Check sheet for the drawn part. Datum: minimum x, y, z corner. Units: mm. Round coordinates to 2 decimals unless told otherwise and drop trailing zeros. Write each loop counter-clockwise with the first axis right and the second up, starting at its lowest first coordinate (ties: lowest second). Pieces come first, ordered by that corner, then holes.
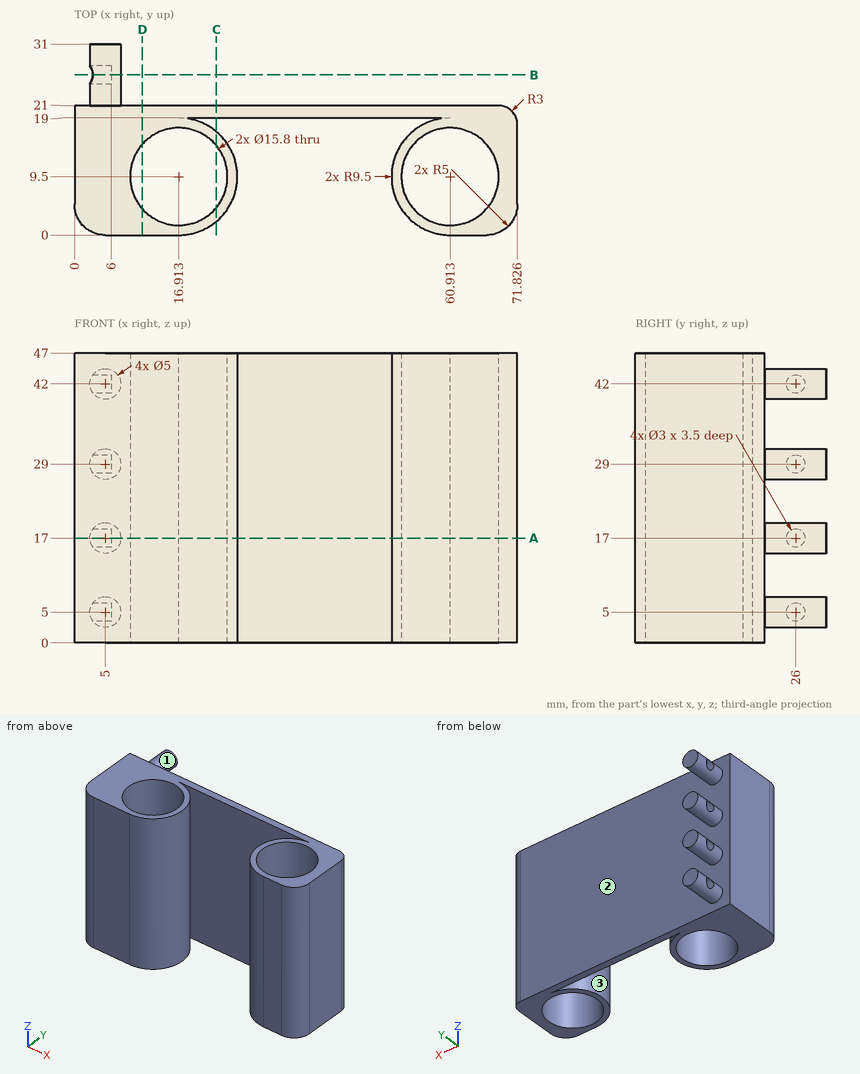
1. Sectioned sample at B-B, the plane y = 26. Enter the section's corners in (x, z).
2. Sectioned sample at D-D, the plane x = 11. Enter the section's corners in (y, z).
3. Release check for a two-part mould opening along Y. For the marked faces 1, 2 and 3 record: released by +Y, released by -Y, zero draft, split by the parting line, or undercut.
4. Scan lines: line 1 along X through (y, z) = (10, 34); line 2 along Y through (x, z) = (56, 24) (1 decimal); line 3 along Y through (x, z) = (5.2, 42). Record each from-to range of solid material in increasing order.
5. Go/stop test with flat-tipped pins: pin 1 (2.5 mm diameter, centred on y = 26, z = 42, fed in from +X); pin 2 (2.5 mm diameter, centred on y = 26, z = 5, fed in from -X); pin 3 (3.5 mm diameter, centred on y = 26, z = 5.5, fed in from -X); pin 4 (6 mm diameter, centred on x = 32, y = 23, fed in from -Z). Record where each tip stops, or that it passes through.
6. Sectioned sample at C-C, the plane x = 23. Enter the section's corners in (y, z).
7. Sectioned sample at A-A, the plane z = 17. Enter the section's corners in (x, y).
Computed values:
1. outline: (3, 3.5) arc R2.5 ccw (long way) to (3, 6.5) - (6, 6.5) - (6, 3.5) - close; (3, 15.5) arc R2.5 ccw (long way) to (3, 18.5) - (6, 18.5) - (6, 15.5) - close; (3, 27.5) arc R2.5 ccw (long way) to (3, 30.5) - (6, 30.5) - (6, 27.5) - close; (3, 40.5) arc R2.5 ccw (long way) to (3, 43.5) - (6, 43.5) - (6, 40.5) - close
2. outline: (0, 0) - (4.26, 0) - (4.26, 47) - (0, 47) - close; (14.74, 0) - (21, 0) - (21, 47) - (14.74, 47) - close
3. face 1: zero draft
3. face 2: released by +Y
3. face 3: undercut
4. line 1: x = 0 to 9.03, 24.8 to 26.4, 51.43 to 53.03, 68.8 to 71.83
4. line 2: y = 1.4 to 3.3, 15.7 to 17.6, 19 to 21
4. line 3: y = 0 to 24.5, 27.5 to 31
5. pin 1: stops at x = 7.5
5. pin 2: stops at x = 6
5. pin 3: stops at x = 2.5
5. pin 4: stops at z = 0
6. outline: (2.21, 0) - (4.46, 0) - (4.46, 47) - (2.21, 47) - close; (14.54, 0) - (16.79, 0) - (16.79, 47) - (14.54, 47) - close; (19, 0) - (21, 0) - (21, 47) - (19, 47) - close
7. outline: (0, 5) arc R5 ccw to (5, 0) - (16.91, 0) arc R9.5 ccw to (16.91, 19) - (60.91, 19) arc R9.5 ccw to (60.91, 0) - (66.83, 0) arc R5 ccw to (71.83, 5) - (71.83, 18) arc R3 ccw to (68.83, 21) - (7.5, 21) - (7.5, 31) - (2.5, 31) - (2.5, 27.5) - (6, 27.5) - (6, 24.5) - (2.5, 24.5) - (2.5, 21) - (0, 21) - close; hole circle Ø15.8 at (16.91, 9.5); hole circle Ø15.8 at (60.91, 9.5)
